from build123d import *


with BuildPart() as part:
    # Sketch2 → Revolve1 (revolve)
    with BuildSketch(Plane(origin=(0, 0, 0), x_dir=(0, 0, -1), z_dir=(1, 0, 0))):
        with BuildLine():
            Line((1255.334291848, 25.4), (1281.455337206, 18.400886991))
            ThreePointArc((1281.455337206, 18.400886991), (1291.638215529, 11.596905223), (1295.574834397, 0))
            Line((1295.574834397, 0), (1255.334291848, 0))
            Line((1255.334291848, 0), (1255.334291848, 22.987))
            Line((1255.334291848, 22.987), (-1255.334291848, 22.987))
            Line((-1255.334291848, 22.987), (-1255.334291848, 0))
            Line((-1255.334291848, 0), (-1295.574834397, 0))
            ThreePointArc((-1295.574834397, 0), (-1291.638215529, 11.596905223), (-1281.455337206, 18.400886991))
            Line((-1281.455337206, 18.400886991), (-1255.334291848, 25.4))
            Line((-1255.334291848, 25.4), (1255.334291848, 25.4))
        make_face()
    revolve(axis=Axis((0, 0, -1295.574834397), (0, 0, 1)))


solid = part.part
Input: part model. Units: mm. Frame: model coordinates. A direction names the side the tool comes from. Coordinates: 2 decimals unless noted, no trailing zeros. Loops run counter-clockwise (first coordinate to the right, second up) from the corner with the lowest first, then second, coordinate; pieces in that order, holes last.
Q1. Contact query for flat-ended pins moving along their axis: pin 1 (14 mm diameter, centred on x = 10, y = -4, fed in from +Z); pin 2 (8 mm diameter, centred on x = -9.5, z = 569, fed in from -Y); pin 3 (8 mm diameter, centred on x = 8, y = -8.5, fed in from +Z). Output: stop coordinate, or through.
Q2. Cut plane A-A (y = 0). Output: boundary loops of the cut face in (x, z), then the cut area to 3 significant figures.
Q3. Set-up query: faces 3 (the face through (-19.38, 12.36, 17.57)), 4 (the face through (24.796, -5.506, -17.575)). Return all of +Z, -Z, +X, -X, +Y, -Y with unobstructed straight access to the full face (end or side cutting, diameter ignored); none if empty.
Q4. Draft query along Y for faces 1 (the face through (-6.13, 19.45, 1274.02)), 2 (the face through (0, 0, 1255.334)). Return one class per face: +Y half, -Y half, draft (parallel to the pull), parting line (faces both ways), or undercut.
Q5. Cut plane C-C (z = 348). Output: boundary loops of the cut face in (x, y).
Q6. Material intervals for line 1 (Y direction, x = 0, z = 6); line 2 (Y direction, x = 1.5, z = -492); line 3 (X direction, y = -3, z = -1092.5), sorted ascending.
Working result:
1. pin 1: stops at z = 1295.2
1. pin 2: stops at y = -24.8
1. pin 3: stops at z = 1293.96
2. outline: (-25.4, -1255.33) - (-18.4, -1281.46) arc R19.05 ccw to (18.4, -1281.46) - (25.4, -1255.33) - (25.4, 1255.33) - (18.4, 1281.46) arc R19.05 ccw to (-18.4, 1281.46) - (-25.4, 1255.33) - close; hole (-22.99, -1255.33) - (22.99, -1255.33) - (22.99, 1255.33) - (-22.99, 1255.33) - close
2. area: 15,200 mm2
3. face 3: none
3. face 4: +Z, -Z
4. face 1: parting line
4. face 2: undercut
5. outline: circle Ø50.8 at (0, 0); hole circle Ø45.97 at (0, 0)
6. line 1: y = -25.4 to -22.99, 22.99 to 25.4
6. line 2: y = -25.36 to -22.94, 22.94 to 25.36
6. line 3: x = -25.22 to -22.79, 22.79 to 25.22
